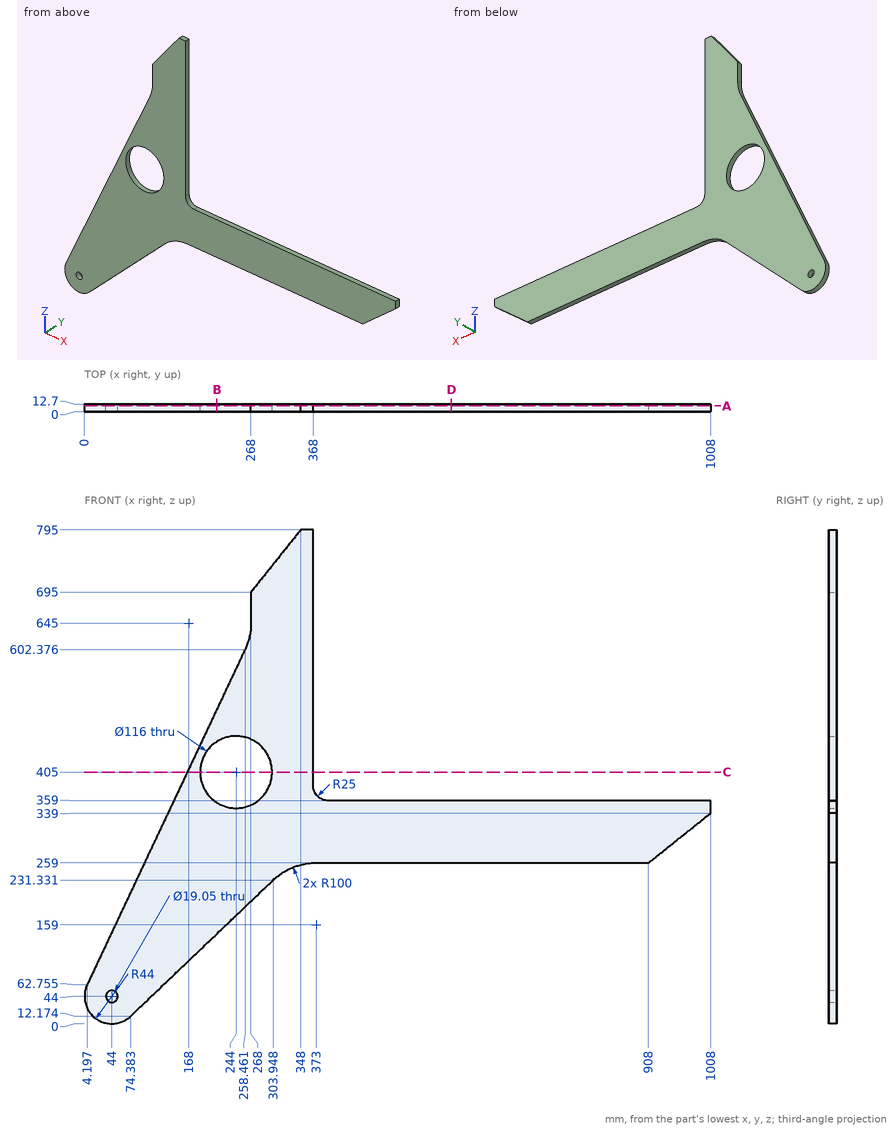
Answer from the drawing. Dimensions are ordinates in mm from the lowest x, y and z of the part. Round coordinates to 2 decimals unless told otherwise and drop trailing zeros. Loops run counter-clockwise (first coordinate to the right, second up) from the corner with the lowest first, then second, coordinate; pieces in that order, holes last.
1) Consider line 1 (Z direction, x = 44, y = 4.25) (1 decimal); line 2 (Z direction, x = 244, y = 5) (1 decimal); line 3 (Z direction, x = 627.5, y = 3). Determine where each line is inside the solid, lowest interval first.
Outcome:
line 1: z = 0 to 34.5, 53.5 to 147.2
line 2: z = 174.1 to 347, 463 to 571.7
line 3: z = 259 to 359
2) A cutting plane is placed at B-B on x = 213. Determine the outline of the cut face in (y, z) (1 decimal), plus the area to 3 significant figures.
Outcome:
outline: (0, 144.5) - (12.7, 144.5) - (12.7, 356) - (0, 356) - close; (0, 454) - (12.7, 454) - (12.7, 505.9) - (0, 505.9) - close
area: 3,340 mm2
3) Given P1, Ø4, axis at y = 7, z = 504.5, coming from the +X side; P2, Ø6, axis at y = 5.5, z = 387, coming from the -X side (1 decimal); P3, Ø2, axis at y = 4, z = 424, coming from the -X side, each flat-ended and moving along its own axis, determine where each tip first touches the part or whether it passes through.
Outcome:
P1: stops at x = 368
P2: stops at x = 155.6
P3: stops at x = 173.94
4) A cutting plane is placed at D-D on x = 590.5. Determine the outline of the cut face in (y, z), plus the area to 3 significant figures.
Outcome:
outline: (0, 259) - (12.7, 259) - (12.7, 359) - (0, 359) - close
area: 1,270 mm2
5) A cutting plane is placed at C-C on z = 405. Determine the outline of the cut face in (x, y), plus the area to 3 significant figures.
Outcome:
outline: (165.46, 0) - (186, 0) - (186, 12.7) - (165.46, 12.7) - close; (302, 0) - (368, 0) - (368, 12.7) - (302, 12.7) - close
area: 1,100 mm2
6) A cutting plane is placed at A-A on y = 9.75. Give the number of separate pieces and of enclosed holes in the cut face, plus the area to 3 significant figures.
Outcome:
separate pieces: 1
enclosed holes: 2
area: 171,000 mm2
